from build123d import *

# Parameters (mm, degrees)
SKETCH_2_W          = 20
SKETCH_2_H          = 4.95
EXTRUDE_1_DEPTH     = 25.6
SKETCH_3_R          = 1.6
CUT_EXTRUDE_1_DEPTH = 5.95
SKETCH_4_W          = 20
SKETCH_4_H          = 4.95
EXTRUDE_2_DEPTH     = 3
CUT_EXTRUDE_2_DEPTH = 3
SKETCH_6_R          = 0.25
CUT_EXTRUDE_3_DEPTH = 3
FILLET_2_R          = 1
SKETCH_7_W          = 2
SKETCH_7_H          = 4.95
CUT_EXTRUDE_4_DEPTH = 29.6
FILLET_3_R          = 3


with BuildPart() as part:
    # 草图2 → 凸台-拉伸1 (new body)
    with BuildSketch(Plane.XY):
        with Locations((10, -2.475)):
            Rectangle(SKETCH_2_W, SKETCH_2_H)
    extrude(amount=EXTRUDE_1_DEPTH)

    # 草图3 → 切除-拉伸1 (cut, through all)
    with BuildSketch(Plane(origin=(0, 0, 0), x_dir=(1, 0, 0), z_dir=(0, 1, 0))):
        with Locations((10, -8.236740591)):
            Circle(SKETCH_3_R)
        with Locations((10, -16.636740591)):
            Circle(SKETCH_3_R)
    extrude(amount=-CUT_EXTRUDE_1_DEPTH, mode=Mode.SUBTRACT)

    # 草图4 → 凸台-拉伸2 (add)
    with BuildSketch(Plane(origin=(0, 0, 0), x_dir=(-1, 0, 0), z_dir=(0, 0, -1))):
        with Locations((-10, -2.475)):
            Rectangle(SKETCH_4_W, SKETCH_4_H)
    extrude(amount=EXTRUDE_2_DEPTH)

    # 草图5 → 切除-拉伸2 (cut)
    with BuildSketch(Plane(origin=(0, 0, -3), x_dir=(-1, 0, 0), z_dir=(0, 0, -1))):
        Polygon((-10, 0), (-7, 0), (-7, -3), (-13, -3), (-13, 0), align=None)
    extrude(amount=-CUT_EXTRUDE_2_DEPTH, mode=Mode.SUBTRACT)

    # 草图6 → 切除-拉伸3 (cut)
    with BuildSketch(Plane(origin=(0, 0, -3), x_dir=(-1, 0, 0), z_dir=(0, 0, -1))):
        with Locations((-7, -3)):
            Circle(SKETCH_6_R)
        with Locations((-13, -3)):
            Circle(SKETCH_6_R)
    extrude(amount=-CUT_EXTRUDE_3_DEPTH, mode=Mode.SUBTRACT)

    # 圆角2
    fillet_2_edges = [part.edges().sort_by_distance(p)[0] for p in [
        (13, 0, -1.5),
        (7, 0, -1.5),
    ]]
    fillet(fillet_2_edges, radius=FILLET_2_R)

    # 草图7 → 切除-拉伸4 (cut, through all)
    with BuildSketch(Plane(origin=(0, 0, -3), x_dir=(-1, 0, 0), z_dir=(0, 0, -1))):
        with Locations((-1, -2.475)):
            Rectangle(SKETCH_7_W, SKETCH_7_H)
        with Locations((-19, -2.475)):
            Rectangle(SKETCH_7_W, SKETCH_7_H)
    extrude(amount=-CUT_EXTRUDE_4_DEPTH, mode=Mode.SUBTRACT)

    # 圆角3
    fillet_3_edges = [part.edges().sort_by_distance(p)[0] for p in [
        (2, -2.475, 25.6),
        (2, -2.475, -3),
        (18, -2.475, 25.6),
        (18, -2.475, -3),
    ]]
    fillet(fillet_3_edges, radius=FILLET_3_R)


solid = part.part
Could you check a few things on this model? Use its own coordinates, in mm. A direction names the side the tool comes from. Round coordinates to 2 decimals unless told otherwise and drop trailing zeros. Loops run counter-clockwise (first coordinate to the right, second up) from the corner with the lowest first, then second, coordinate; pieces in that order, holes last. Notation, with made-up numbers: (54.25, -19.5) -> (79.25, -19.5) arc R17 ccw to (79.25, 10.5) -> close; hole circle Ø6 at (-21, -6.75). An arc over 180 degrees is marked (long way). Use CSV: the item, a comma, the result in double quotes.
(1) For faces 1 (the cylindrical face through (6.699, -0.285, -1.479)), 2 (the flat face through (10, -4.95, 12)), which set-ups out of +Z, -Z, +X, -X, +Y, -Y let a thin tool reach every point of the face, with its end or its side?
Return value:
face 1,"-Z, +Y"
face 2,"+Z, -Z, +X, -X, -Y"
(2) Suppose I cut it at D-D on y = -2.25. Write out the boundary of the cut face in (x, z).
Return value:
outline,"(2, 0) arc R3 ccw to (5, -3) -> (7, -3) -> (7, 0) -> (13, 0) -> (13, -3) -> (15, -3) arc R3 ccw to (18, 0) -> (18, 22.6) arc R3 ccw to (15, 25.6) -> (5, 25.6) arc R3 ccw to (2, 22.6) -> close; hole circle Ø3.2 at (10, 8.24); hole circle Ø3.2 at (10, 16.64)"
(3) Will these pins go through, and if not, where does the flat tip stop? pin 1 Ø1 at (x, y) = (8, -1) entering from -Z; pin 2 Ø4 at (x, z) = (10, 8.24) entering from -Y; pin 3 Ø1.5 at (x, z) = (10.5, -2) entering from +Y; pin 4 Ø0.9 at (y, z) = (-2, -1) entering from -X.
Return value:
pin 1,"stops at z = 0"
pin 2,"stops at y = -4.95"
pin 3,"stops at y = -3"
pin 4,"stops at x = 2.05"
(4) If we mould it in two halves opening along X, with no side actions, what happens to faces 3 (the cylindrical face through (2.9, -2.51, 24.74)), 4 (the cylindrical face through (17.1, -2.44, -2.14)), 5 (the flat face through (10, -3, -2))? For each: +X half, -X half, draft (parallel to the pull), parting line (faces both ways), or undercut.
Return value:
face 3,"-X half"
face 4,"+X half"
face 5,"undercut"
(5) If I drill on probe 1 along Z at (x, y) = (10, -3.4); probe 2 along Z at (x, y) = (10, -2.3); probe 3 along X at (y, z) = (-0.85, 16.5), over which ranges is the centre line in solid material (lowest first)? Write a range as [from, to].
Return value:
probe 1,"z = [-3, 6.64], [9.84, 15.04], [18.24, 25.6]"
probe 2,"z = [0, 6.64], [9.84, 15.04], [18.24, 25.6]"
probe 3,"x = [2, 8.41], [11.59, 18]"
(6) Suppose I cut it at C-C on y = -0.7. Write out the boundary of the cut face in (x, z), plus the area to 3 significant figures.
Return value:
outline,"(2, 0) arc R3 ccw to (5, -3) -> (6.95, -3) -> (6.95, 0) -> (13.05, 0) -> (13.05, -3) -> (15, -3) arc R3 ccw to (18, 0) -> (18, 22.6) arc R3 ccw to (15, 25.6) -> (5, 25.6) arc R3 ccw to (2, 22.6) -> close; hole circle Ø3.2 at (10, 8.24); hole circle Ø3.2 at (10, 16.64)"
area,"416 mm²"
(7) Suppose I cut it at B-B on z = 16.25. Write out the boundary of the cut face in (x, y), plus the area to 3 significant figures.
Return value:
outline,"(2, -4.95) -> (8.45, -4.95) -> (8.45, 0) -> (2, 0) -> close; (11.55, -4.95) -> (18, -4.95) -> (18, 0) -> (11.55, 0) -> close"
area,"63.8 mm²"
(8) Suppose I cut it at A-A on x = 10. Write out the boundary of the cut face in (y, z), plus the area to 3 significant figures.
Return value:
outline,"(-4.95, -3) -> (-3, -3) -> (-3, 0) -> (0, 0) -> (0, 6.64) -> (-4.95, 6.64) -> close; (-4.95, 9.84) -> (0, 9.84) -> (0, 15.04) -> (-4.95, 15.04) -> close; (-4.95, 18.24) -> (0, 18.24) -> (0, 25.6) -> (-4.95, 25.6) -> close"
area,"101 mm²"
